from build123d import *

# Parameters (mm, degrees)
SKETCH1_R           = 1.55
SKETCH1_R_2         = 5
SKETCH1_R_3         = 6
BOSS_EXTRUDE1_DEPTH = 3
FILLET1_R           = 3
SKETCH_3_R          = 2.1
CUT_EXTRUDE_1_DEPTH = 10


with BuildPart() as part:
    # Sketch1 → Boss-Extrude1 (new body)
    with BuildSketch(Plane(origin=(0, 0, 0), x_dir=(1, 0, 0), z_dir=(0, 1, 0))):
        Polygon((-62, 19), (62, 19), (62, 13), (59, 13), (59, -13), (62, -13), (62, -19), (-62, -19), (-62, -13), (-59, -13), (-59, 13), (-62, 13), align=None)
        with Locations(Location((55.5, 11, 0), (0, 0, 270))):
            Circle(SKETCH1_R, mode=Mode.SUBTRACT)
        with Locations(Location((-55.5, 11, 0), (0, 0, 90))):
            Circle(SKETCH1_R, mode=Mode.SUBTRACT)
        with Locations(Location((-55.5, -11, 0), (0, 0, 270))):
            Circle(SKETCH1_R, mode=Mode.SUBTRACT)
        with Locations(Location((55.5, -11, 0), (0, 0, 90))):
            Circle(SKETCH1_R, mode=Mode.SUBTRACT)
        with Locations(Location((0, 0, 0), (0, 0, 270))):
            Circle(SKETCH1_R_2, mode=Mode.SUBTRACT)
        with Locations(Location((20, 0, 0), (0, 0, 270))):
            Circle(SKETCH1_R, mode=Mode.SUBTRACT)
        with Locations(Location((-20, 0, 0), (0, 0, 90))):
            Circle(SKETCH1_R, mode=Mode.SUBTRACT)
        with Locations(Location((35, 0, 0), (0, 0, 270))):
            Circle(SKETCH1_R_3, mode=Mode.SUBTRACT)
        with Locations(Location((-35, 0, 0), (0, 0, 90))):
            Circle(SKETCH1_R_3, mode=Mode.SUBTRACT)
        with Locations(Location((47, 9, 0), (0, 0, 270))):
            Circle(SKETCH1_R, mode=Mode.SUBTRACT)
        with Locations(Location((47, -9, 0), (0, 0, 90))):
            Circle(SKETCH1_R, mode=Mode.SUBTRACT)
        with Locations(Location((-47, -9, 0), (0, 0, 270))):
            Circle(SKETCH1_R, mode=Mode.SUBTRACT)
        with Locations(Location((-47, 9, 0), (0, 0, 90))):
            Circle(SKETCH1_R, mode=Mode.SUBTRACT)
    extrude(amount=BOSS_EXTRUDE1_DEPTH)

    # Fillet1
    fillet1_edges = [part.edges().sort_by_distance(p)[0] for p in [
        (-62, 1.5, -19),
        (-62, 1.5, -13),
        (-62, 1.5, 13),
        (-62, 1.5, 19),
        (62, 1.5, 19),
        (62, 1.5, 13),
        (62, 1.5, -13),
        (62, 1.5, -19),
    ]]
    fillet(fillet1_edges, radius=FILLET1_R - 0.0001)  # a hair under: the kernel refuses the full size

    # 草图3 → 切除-拉伸1 (cut)
    with BuildSketch(Plane.XZ):
        with Locations(Location((-30.748546153, -13.88500521, 0), (0, 0, 270))):
            Circle(SKETCH_3_R)
        with Locations(Location((-30.748546153, 16.11499479, 0), (0, 0, 270))):
            Circle(SKETCH_3_R)
    extrude(amount=-CUT_EXTRUDE_1_DEPTH, mode=Mode.SUBTRACT)


solid = part.part
Geometry check sheet. Reference: the model listing, model coordinates, mm. A direction names the side the tool comes from. Round coordinates to 2 decimals unless told otherwise and drop trailing zeros. Order: outer loops, then holes, each group sorted by start corner. A loop starts at its lowest first (then second) coordinate and runs counter-clockwise, first axis right, second up. Notation, with made-up numbers: M 73.25,18 L 86.25,18 A7 ccw 86.25,22 Z; hole C -21.5,11.25 d10. An arc over 180 degrees is marked long. Write each question's results on one line, items separated by ' | '. Start each with the question number.
1. Draft check along Z on faces 1 (the face through (61.1, 1.52, -18.14)), 2 (the face through (-32.8, 1.48, -13.43)), 3 (the face through (1, 0, -9)). Enter one of: pulls with the +Z half, pulls with the -Z half, needs draft (parallel to the pull), parting line crosses it, or undercut.
2. Go/stop test with flat-tipped pins: P1, Ø1, axis at y = 1.5, z = 2.5, coming from the -X side; P2, Ø1.5, axis at y = 1, z = -12.5, coming from the -X side. Record where each tip stops, or that it passes through.
3. Cross-section at B-B on x = 0. Record the boundary of the cut face in (y, z).
4. Set-up check for faces 4 (the face through (59, 1, 0)), 5 (the face through (29.143, 1.479, -1.301)), 6 (the face through (-59, 1, 0)): record each of +Z, -Z, +X, -X, +Y, -Y from which the full face is reachable in a straight line by a thin tool's end or side.
5. Cross-section at A-A on x = -47. Record the boundary of the cut face in (y, z).
6. Cross-section at C-C on x = -20. Record the boundary of the cut face in (y, z), plus the area to 3 significant figures.
7. Material ranges on L1, parallel to X at y = 0.9, z = -9; L2, parallel to X at y = 1.35, z = 0; L3, parallel to X at y = 0.9, z = 11, recorded low to high. Write a range as from..to.
8. Cross-section at D-D on y = 0.6. Give the number of separate pieces and of enclosed holes in the cut face, plus the area to 3 significant figures.
Resolved:
1) face 1: pulls with the -Z half | face 2: undercut | face 3: needs draft
2) P1: x = -59 | P2: x = -60.2
3) outline: M 0,-19 L 3,-19 L 3,-5 L 0,-5 Z; M 0,5 L 3,5 L 3,19 L 0,19 Z
4) face 4: +X, +Y, -Y | face 5: +Y, -Y | face 6: -X, +Y, -Y
5) outline: M 0,-19 L 3,-19 L 3,-10.55 L 0,-10.55 Z; M 0,-7.45 L 3,-7.45 L 3,7.45 L 0,7.45 Z; M 0,10.55 L 3,10.55 L 3,19 L 0,19 Z
6) outline: M 0,-19 L 3,-19 L 3,-1.55 L 0,-1.55 Z; M 0,1.55 L 3,1.55 L 3,19 L 0,19 Z | area: 105 mm2
7) L1: -59..-48.55, -45.45..45.45, 48.55..59 | L2: -59..-41, -29..-21.55, -18.45..-5, 5..18.45, 21.55..29, 41..59 | L3: -59..-57.05, -53.95..53.95, 57.05..59
8) separate pieces: 1 | enclosed holes: 15 | area: 4,130 mm2
